Read the model definition and answer for the solid it produces. Units are mm, in the model's axes. A direction names the side the tool comes from. Give positions to 0.01 mm unless a question says otherwise; leave off trailing zeros. Order: outer loops, then holes, each group sorted by start corner. A loop starts at its lowest first (then second) coordinate and runs counter-clockwise, first axis right, second up. Notation, with made-up numbers: (-2, 43.5) - (33, 43.5) arc R19 ccw to (33, 58.5) - close; hole circle Ø11 at (9, 36). An arc over 180 degrees is marked (long way). Write each question's results on one line, items separated by ' | '.
Autodesk Inventor part; units mm, degrees
ref_plane "YZ-Ebene" through (0, 0, 0) normal (1, 0, 0) x (0, 1, 0)
ref_plane "XZ-Ebene" through (0, 0, 0) normal (0, 1, 0) x (-1, 0, 0)
ref_plane "XY-Ebene" through (0, 0, 0) normal (0, 0, 1) x (1, 0, 0)
sketch "Skizze1" plane through (0, 0, 0) normal (0, 0, 1) x (1, 0, 0)
  line L0 (-6.24, 0) -> (1.04, 0)
  line L1 (0, -0.5) -> (0, 3)
  line L2 (-5.2, 0) -> (-5.2, 2)
  line L3 (-5.2, 2) -> (-3.2, 2.5)
  line L4 (-3.2, 2.5) -> (-1.6, 2.5)
  line L5 (-1.6, 2.5) -> (-1.6, 1.5)
  line L6 (-1.6, 1.5) -> (-4, 1.5)
  line L7 (-4, 1.5) -> (-4, 0)
  point P0 (0, 0)
  dimension "d3" = 3.2
  dimension "d4" = 6.4
  dimension "d5" = 8
  dimension "d6" = 10.4
  dimension "d7" = 2
  dimension "d8" = 2.5
  dimension "d9" = 1.5
revolve "Umdrehung1" add sketch "Skizze1" angle 360 about axis through (0, -10, 0) along (0, 1, 0)
properties part number "Deckel_ra8846s" material "Stahl"
(1) The mould has two halves that part along X. Classify faces 1 (the face through (1.27, 1.99, 0.97)), 2 (the face through (-3, 0, -3)), 3 (the face through (0.677, 1.014, 5.156)): pulls with the +X half, pulls with the -X half, needs draft (parallel to the pull), parting line crosses it, or undercut.
Conclusion:
face 1: undercut | face 2: needs draft | face 3: parting line crosses it
(2) Section B-B (x = 0) is taken. Give the vertices of the cut face in (y, z).
Conclusion:
outline: (0, -5.2) - (2, -5.2) - (2.5, -3.2) - (2.5, -1.6) - (1.5, -1.6) - (1.5, -4) - (0, -4) - close; (0, 4) - (1.5, 4) - (1.5, 1.6) - (2.5, 1.6) - (2.5, 3.2) - (2, 5.2) - (0, 5.2) - close
(3) Section D-D (y = 0.55) is taken. Give the vertices of the cut face in (x, z), plus the area to 3 significant figures.
Conclusion:
outline: circle Ø10.4 at (0, 0); hole circle Ø8 at (0, 0) | area: 34.7 mm^2
(4) Each of these flat-tipped pins is pushed along its axis until it touches: pin 1 (1.5 mm diameter, centred on y = 0.5, z = -3, fed in from -X); pin 2 (1.5 mm diameter, centred on x = 2, y = 0.5, fed in from +Z); pin 3 (1.5 mm diameter, centred on x = -3, z = 2, fed in from +Y); pin 4 (5 mm diameter, centred on x = 0, z = 0, fed in from -Y). Where does it stop, or does it pass through?
Conclusion:
pin 1: x = -4.69 | pin 2: z = 5.05 | pin 3: y = 2.5 | pin 4: y = 1.5
(5) Section C-C (y = 2.15) is taken. Give the vertices of the cut face in (x, z), plus the area to 3 significant figures.
Conclusion:
outline: circle Ø9.2 at (0, 0); hole circle Ø3.2 at (0, 0) | area: 58.4 mm^2
(6) For faces 4 (the face through (0.867, 0.74, 3.905)), 5 (the face through (-1.4, 2.5, -1.4)), determine the directions among +Z, -Z, +X, -X, +Y, -Y from which every point of the face is accessible in a straight line to the end or side of a thin tool.
Conclusion:
face 4: -Y | face 5: +Z, -Z, +X, -X, +Y
(7) Consider probe 1 along Z at (x, y) = (0, 1.15); probe 2 along Z at (x, y) = (0, 1.7); probe 3 along Y at (x, z) = (2, -2.25). Determine where each line is inside the solid, lowest interval first. Write a range as [from, to].
Conclusion:
probe 1: [-5.2, -4], [4, 5.2] | probe 2: [-5.2, -1.6], [1.6, 5.2] | probe 3: [1.5, 2.5]
(8) Section A-A (z = 0) is taken. Give the vertices of the cut face in (x, y).
Conclusion:
outline: (-5.2, 0) - (-4, 0) - (-4, 1.5) - (-1.6, 1.5) - (-1.6, 2.5) - (-3.2, 2.5) - (-5.2, 2) - close; (1.6, 1.5) - (4, 1.5) - (4, 0) - (5.2, 0) - (5.2, 2) - (3.2, 2.5) - (1.6, 2.5) - close
